from build123d import *

# Parameters (mm, degrees)
BOSS_EXTRUDE2_DEPTH = 20
SHELL2_T            = -1
SKETCH2_R           = 1.5
BOSS_EXTRUDE4_DEPTH = 2


with BuildPart() as part:
    # Sketch1 → Boss-Extrude2 (new body)
    with BuildSketch(Plane.XY):
        Polygon((-3.474068414, 12.465208849), (-23.683257598, 29), (-37, 29), (-37, -29), (-23.683257598, -29), (-3.474068414, -12.465208849), (9.474068414, -12.465208849), (29.683257598, -29), (37, -29), (37, 29), (29.683257598, 29), (9.474068414, 12.465208849), align=None)
        Polygon((-33, 19.559028944), (-16.790810816, 6.296965066), (-16.790810816, -4.296965066), (-33, -17.559028944), align=None, mode=Mode.SUBTRACT)
        Polygon((16.790810816, 8.296965066), (33, 21.559028944), (33, -15.559028944), (16.790810816, -2.296965066), align=None, mode=Mode.SUBTRACT)
    extrude(amount=BOSS_EXTRUDE2_DEPTH)

    # Shell2
    shell2_openings = [part.faces().sort_by_distance(p)[0] for p in [
        (24.895405408, -8.927997005, 10),
        (33, 3, 10),
        (24.895405408, 14.927997005, 10),
        (16.790810816, 3, 10),
        (-16.790810816, 1, 10),
        (-24.895405408, 12.927997005, 10),
        (-33, 1, 10),
        (-24.895405408, -10.927997005, 10),
        (33.341628799, -29, 10),
        (19.578663006, -20.732604425, 10),
        (3, -12.465208849, 10),
        (-13.578663006, -20.732604425, 10),
        (-30.341628799, -29, 10),
        (-13.578663006, 20.732604425, 10),
        (3, 12.465208849, 10),
        (19.578663006, 20.732604425, 10),
    ]]
    offset(amount=SHELL2_T, openings=shell2_openings, kind=Kind.INTERSECTION)

    # Sketch2 → Boss-Extrude4 (add)
    with BuildSketch(Plane.XY):
        with BuildLine():
            Line((-39.5, -1.865744817), (-37, -1.865744817))
            Line((-37, -1.865744817), (-37, 3.134255183))
            Line((-37, 3.134255183), (-39.5, 3.134255183))
            ThreePointArc((-39.5, 3.134255183), (-42, 0.634255183), (-39.5, -1.865744817))
        make_face()
        with Locations((-39.5, 0.634255183)):
            Circle(SKETCH2_R, mode=Mode.SUBTRACT)
        with BuildLine():
            Line((39.5, 3.134255183), (37, 3.134255183))
            Line((37, 3.134255183), (37, -1.865744817))
            Line((37, -1.865744817), (39.5, -1.865744817))
            ThreePointArc((39.5, -1.865744817), (42, 0.634255183), (39.5, 3.134255183))
        make_face()
        with Locations((39.5, 0.634255183)):
            Circle(SKETCH2_R, mode=Mode.SUBTRACT)
    extrude(amount=BOSS_EXTRUDE4_DEPTH)


solid = part.part
Geometry: final body of the model. Coordinates: model frame, mm. A direction names the side the tool comes from. Round coordinates to 2 decimals unless told otherwise and drop trailing zeros. Loops run counter-clockwise (first coordinate to the right, second up) from the corner with the lowest first, then second, coordinate; pieces in that order, holes last. Notation, with made-up numbers: M 66,51.25 L 101,51.25 A20 cw 101,64.25 Z; hole C -11.5,25.5 d11. An arc over 180 degrees is marked long. Put each result on its own line as item: value. Start each with the question number.
(1) Section query B-B (x = 7.5). Return loops of the section in (y, z).
(2) Material intervals for line 1 along X through (y, z) = (-11.5, 15.75); line 2 along Y through (x, z) = (39.5, 1.3); line 3 along Z through (x, y) = (-34, -15.5), sorted ascending. Write a range as [from, to].
(3) Set-up query: faces 4 (the face through (-1, 0, 1)), 5 (the face through (19.44, -20.62, 19.49)), 6 (the face through (24.782, 14.835, 19.493)). Return all of +Z, -Z, +X, -X, +Y, -Y with unobstructed straight access to the full face (end or side cutting, diameter ignored); none if empty.
(4) Section query D-D (x = 18). Return loops of the section in (y, z).
(5) Section query C-C (y = -19.5). Return loops of the section in (x, z), then the cut area to 3 significant figures.
(6) Contact query for flat-ended pins moving along their axis: pin 1 Ø6 at (y, z) = (11.5, 5.5) entering from +X; pin 2 Ø0.5 at (x, z) = (1.5, 19.5) entering from -Y; pin 3 Ø1 at (x, z) = (38.5, 1.5) entering from +Y. Output: stop coordinate, or through.
(7) Draft query along X for faces 1 (the face through (19.44, -20.62, 0.49)), 2 (the face through (-29, 28, 10)), 3 (the face through (-38, 3.134, 1)). Return one class per face: +X half, -X half, draft (parallel to the pull), parting line (faces both ways), or undercut.
(8) Section query A-A (z = 5.75). Return loops of the section in (x, y).
Findings below:
1. outline: M -12.47,0 L 12.47,0 L 12.47,1 L -12.47,1 Z; M -12.47,19 L 12.47,19 L 12.47,20 L -12.47,20 Z
2. line 1: x = [-37, -36], [36, 37]
2. line 2: y = [-1.87, -0.87], [2.13, 3.13]
2. line 3: z = [0, 1], [19, 20]
3. face 4: -Y
3. face 5: +Z, -Z, -Y
3. face 6: +Z, -Z
4. outline: M -19.44,0 L -3.29,0 L -3.29,1 L -19.44,1 Z; M -19.44,19 L -3.29,19 L -3.29,20 L -19.44,20 Z; M 9.29,0 L 19.44,0 L 19.44,1 L 9.29,1 Z; M 9.29,19 L 19.44,19 L 19.44,20 L 9.29,20 Z
5. outline: M -37,0 L -12.07,0 L -12.07,1 L -36,1 L -36,19 L -12.07,19 L -12.07,20 L -37,20 Z; M 18.07,0 L 37,0 L 37,20 L 18.07,20 L 18.07,19 L 36,19 L 36,1 L 18.07,1 Z
5. area: 124 mm2
6. pin 1: stops at x = 37
6. pin 2: stops at y = -12.47
6. pin 3: stops at y = 3.13
7. face 1: undercut
7. face 2: undercut
7. face 3: draft
8. outline: M -37,-29 L -36,-29 L -36,28 L -22.46,28 L -23.68,29 L -37,29 Z; M 28.46,28 L 36,28 L 36,-29 L 37,-29 L 37,29 L 29.68,29 Z
